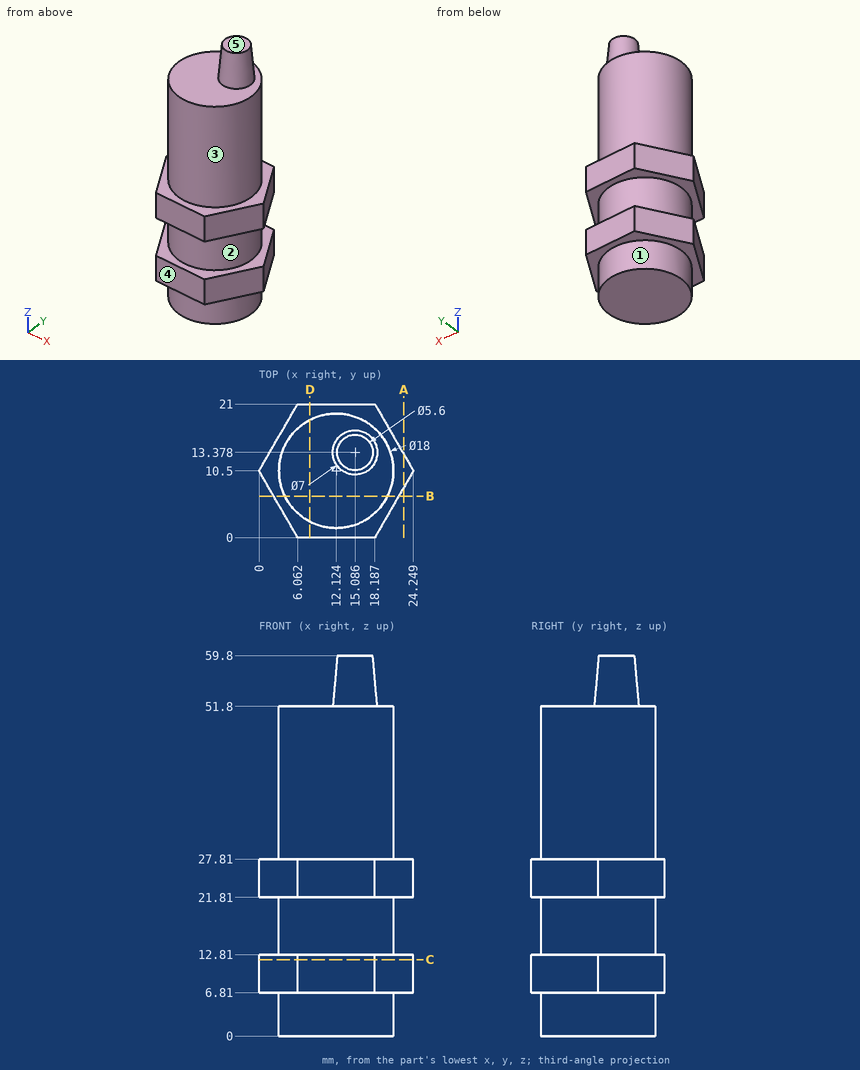
Could you check a few things on this drawing? It's one solid part, dimensions in mm from its lowest x, y, z. A direction names the side the tool comes from. Coordinates: 2 decimals unless noted, no trailing zeros. Loops run counter-clockwise (first coordinate to the right, second up) from the corner with the lowest first, then second, coordinate; pieces in that order, holes last.
1. I need wall thicknesses on L1, parallel to Z at x = 3, y = 9; L2, parallel to Z at x = 18, y = 16.75; L3, parallel to X at y = 10, z = 17.5. Which ranges of each line are inside material? Lowest first, please.
2. For the marked faces 1, 2, 3, 4 and 5, which set-ups out of +Z, -Z, +X, -X, +Y, -Y let a thin tool reach every point of the face, with its end or its side?
3. Imagine slicing it at D-D (x = 8). Please give me the cut outline in (y, z).
4. Imagine slicing it at A-A (x = 22.75). Please give me the cut outline in (y, z) (1 decimal).
5. Imagine slicing it at B-B (y = 6.5). Please give me the cut outline in (x, z), and give its area (3 significant figures).
6. For P1, Ø5, axis at x = 15.5, z = 46.5, coming from the +Y side; P2, Ø1.5, axis at x = 12.5, z = 33.5, coming from the -Y side; P3, Ø3, axis at y = 3.5, z = 23, coming from the -X side (1 decimal), each with a flat end and sliding along its axis, tell me the tip position at first contact or that it passes through.
7. Imagine slicing it at C-C (z = 12). Please give me the cut outline in (x, y), and give its area (3 significant figures).
Computed values:
1. L1: z = 6.81 to 12.81, 21.81 to 27.81
1. L2: z = 0 to 51.8
1. L3: x = 3.14 to 21.11
2. face 1: -Z
2. face 2: none
2. face 3: +Z
2. face 4: +Z, -Z, +X, -X, -Y
2. face 5: +Z, +X, -X, +Y, -Y
3. outline: (0, 6.81) - (2.5, 6.81) - (2.5, 0) - (18.5, 0) - (18.5, 6.81) - (21, 6.81) - (21, 12.81) - (18.5, 12.81) - (18.5, 21.81) - (21, 21.81) - (21, 27.81) - (18.5, 27.81) - (18.5, 51.8) - (2.5, 51.8) - (2.5, 27.81) - (0, 27.81) - (0, 21.81) - (2.5, 21.81) - (2.5, 12.81) - (0, 12.81) - close
4. outline: (7.9, 6.8) - (13.1, 6.8) - (13.1, 12.8) - (7.9, 12.8) - close; (7.9, 21.8) - (13.1, 21.8) - (13.1, 27.8) - (7.9, 27.8) - close
5. outline: (2.31, 6.81) - (4.06, 6.81) - (4.06, 0) - (20.19, 0) - (20.19, 6.81) - (21.94, 6.81) - (21.94, 12.81) - (20.19, 12.81) - (20.19, 21.81) - (21.94, 21.81) - (21.94, 27.81) - (20.19, 27.81) - (20.19, 51.8) - (4.06, 51.8) - (4.06, 27.81) - (2.31, 27.81) - (2.31, 21.81) - (4.06, 21.81) - (4.06, 12.81) - (2.31, 12.81) - close
5. area: 877 mm2
6. P1: stops at y = 19.46
6. P2: stops at y = 1.5
6. P3: stops at x = 3.2
7. outline: (0, 10.5) - (6.06, 0) - (18.19, 0) - (24.25, 10.5) - (18.19, 21) - (6.06, 21) - close
7. area: 382 mm2
